```python
from build123d import *

# Parameters (mm, degrees)
F0_R     = 14
F1_DEPTH = 25
F3_R     = 7.5
F4_DEPTH = 50


# Not quite as in the source:
# - a fillet or chamfer that OpenCascade refuses, or shapes differently, is made with other operations: its cross-section is extruded or revolved along the edge and cut away or added


with BuildPart() as f1:
    # F0 (on Top) → F1 (new body)
    with BuildSketch(Plane.XY):
        Circle(F0_R)
    extrude(amount=F1_DEPTH)

    # F2: chamfer of 8 x 35 on 1 edges, made by hand

    # F2_s1 → F2_t2 (revolve, cut)
    with BuildSketch(Plane.XZ):
        Polygon((14, -10), (6, 25), (14, 25), align=None)
    revolve(axis=Axis((0, 0, 25), (0, 0, 1)), mode=Mode.SUBTRACT)

    # F3 (on face) → F4 (join)
    with BuildSketch(Plane(origin=(0, 0, 0), x_dir=(1, 0, 0), z_dir=(0, 0, -1))):
        Circle(F3_R)
    extrude(amount=F4_DEPTH)


solid = f1.part
```
Verification items for the finished model (mm, model axes). A direction names the side the tool comes from. Round coordinates to 2 decimals unless told otherwise and drop trailing zeros. Write each loop counter-clockwise with the first axis right and the second up, starting at its lowest first coordinate (ties: lowest second). Pieces come first, ordered by that corner, then holes. Notation, with made-up numbers: (19.5, 65.25) -> (24.5, 65.25) arc R33 ccw to (24.5, 97.25) -> close; hole circle Ø11 at (81, 80.5). An arc over 180 degrees is marked (long way). Write each question's results on one line, items separated by ' | '.
Q1. Sectioned sample at A-A, the plane y = 0. Record the boundary of the cut face in (x, z).
Derived:
outline: (-11.71, 0) -> (-7.5, 0) -> (-7.5, -50) -> (7.5, -50) -> (7.5, 0) -> (11.71, 0) -> (6, 25) -> (-6, 25) -> close
Q2. Thickness scan on probe 1 along Y at (x, z) = (-4.5, 13); probe 2 along X at (y, z) = (-0.75, -33); probe 3 along X at (y, z) = (3.5, -5.5). Record the ranges inside material, lowest first.
Derived:
probe 1: y = -7.5 to 7.5 | probe 2: x = -7.46 to 7.46 | probe 3: x = -6.63 to 6.63
Q3. Go/stop test with flat-tipped pins: pin 1 Ø5 at (x, z) = (-0.5, -18) entering from -Y; pin 2 Ø4 at (x, z) = (-6, -32.5) entering from -Y; pin 3 Ø1 at (x, y) = (-8.5, -6) entering from -Z. Record where each tip stops, or that it passes through.
Derived:
pin 1: stops at y = -7.5 | pin 2: stops at y = -6.34 | pin 3: stops at z = 0
Q4. Access from +Z, -Z, +X, -X, +Y, -Y to the whole of each face (thin tool, end or side, straight path). Record for faces 1 (the face through (0, -8, 0)), 2 (the face through (-6.493, -4.979, 15.453)).
Derived:
face 1: -Z | face 2: +Z
Q5. Sectioned sample at C-C, the plane z = -31.5. Record the boundary of the cut face in (x, y), and give its area (3 significant figures).
Derived:
outline: circle Ø15 at (0, 0) | area: 177 mm²
